The listing builds one solid part. Answer for the finished solid, in the listing's coordinates (mm). Face numbers are marked on the shaded views. A direction names the side the tool comes from. Coordinates: 2 decimals unless noted, no trailing zeros. Order: outer loops, then holes, each group sorted by start corner. A loop starts at its lowest first (then second) coordinate and runs counter-clockwise, first axis right, second up. Notation, with made-up numbers: (-18.75, -26.75) - (36.25, -26.75) arc R22 ccw to (36.25, 10.25) - close; hole circle Ø11 at (14, 81). An arc over 180 degrees is marked (long way). Use one line per item in the form item = value. Start each with the question number.
Item 1: Section A-A, the plane x = 250.5 is taken. Write down the section's boundary in (y, z).
Item 2: Section C-C, the plane x = -10 is taken. Write down the section's boundary in (y, z), and give its area (3 significant figures).
Item 3: Section D-D, the plane z = 117 is taken. Write down the section's boundary in (x, y), and give its area (3 significant figures).
Item 4: A tool of negligible diameter and unlimited length cuts with its end or side. For the marked faces 1 and 2, from which of +Z, -Z, +X, -X, +Y, -Y can it reach the whole face along a straight path? Write none if from no direction.
Item 5: Each of these flat-tipped pins is pushed along its axis until it touches: pin 1 Ø10 at (y, z) = (631.5, 111) entering from -X; pin 2 Ø8 at (x, z) = (366, 13.5) entering from -Y; pin 3 Ø6 at (y, z) = (89.5, 49.5) entering from -X. Where does it stop, or does it pass through?
Item 6: Section B-B, the plane z = 54.5 is taken. Write down the section's boundary in (x, y).
Item 7: The mould has two halves that part along Y. Classify the marked faces 3, 4 and 5: released by +Y, released by -Y, zero draft, split by the parting line, or undercut.
Item 8: Consider line 1 along Y through (x, z) = (99, 37.5); line 2 along X through (y, z) = (195, 49); line 3 along X through (y, z) = (688.5, 42.5). Determine where each line is inside the solid, lowest interval first. Write a range as [from, to].
Autodesk Inventor part; units mm, degrees
ref_plane "YZ Plane" through (0, 0, 0) normal (1, 0, 0) x (0, 1, 0)
ref_plane "XZ Plane" through (0, 0, 0) normal (0, 1, 0) x (-1, 0, 0)
ref_plane "XY Plane" through (0, 0, 0) normal (0, 0, 1) x (1, 0, 0)
sketch "Sketch1" plane through (0, 0, 0) normal (0, 0, 1) x (1, 0, 0)
  line L0 (0, 0) -> (351.6706, 0)
  line L1 (-103.5647, 179.3793) -> (0, 0)
  line L2 (351.6706, 0) -> (455.2353, 179.3793)
  line L3 (455.2353, 179.3793) -> (455.2353, 534.9793)
  line L4 (-103.5647, 534.9793) -> (-103.5647, 179.3793)
  line L5 (0, 714.3586) -> (-103.5647, 534.9793)
  line L6 (356.3091, 714.3586) -> (0, 714.3586)
  line L7 (455.2353, 534.9793) -> (356.3091, 714.3586)
  line L8 (-103.5647, 179.3793) -> (-192.4647, 179.3793) construction
  line L9 (-51.7823, 89.6897) -> (-128.772, 45.2397) construction
  line L10 (-128.772, 45.2397) -> (-51.7823, -88.9)
  line L11 (-51.7823, -88.9) -> (0, -88.9)
  line L12 (178.1545, -88.9) -> (178.1545, 714.3586) construction
  line L13 (178.1545, -88.9) -> (0, -88.9)
  line L14 (-128.772, 45.2397) -> (-192.4647, 156.2119)
  line L15 (-192.4647, 156.2119) -> (-192.4647, 179.3793)
  line L16 (178.1545, 714.3586) -> (178.1545, 803.2586) construction
  line L17 (-51.7823, 624.669) -> (-128.772, 669.119) construction
  line L18 (-192.4647, 179.3793) -> (-192.4647, 558.8)
  line L19 (-192.4647, 558.8) -> (-128.772, 669.119)
  line L20 (178.1545, 803.2586) -> (-51.3264, 803.2586)
  line L21 (-51.3264, 803.2586) -> (-128.772, 669.119)
  line L22 (485.0811, 45.2397) -> (408.0914, -88.9)
  line L23 (178.1545, -88.9) -> (356.3091, -88.9)
  line L24 (485.0811, 45.2397) -> (548.7738, 156.2119)
  line L25 (548.7738, 156.2119) -> (548.7738, 179.3793)
  line L26 (408.0914, 624.669) -> (485.0811, 669.119) construction
  line L27 (548.7738, 179.3793) -> (548.7738, 558.8)
  line L28 (548.7738, 558.8) -> (485.0811, 669.119)
  line L29 (178.1545, 803.2586) -> (407.6355, 803.2586)
  line L30 (407.6355, 803.2586) -> (485.0811, 669.119)
  line L31 (408.0914, -88.9) -> (356.3091, -88.9)
  point P0 (175.8353, 357.1793)
  dimension "d0" = 88.9
  dimension "d1" = 88.9
  dimension "d2" = 88.9
  dimension "d3" = 88.9
  dimension "d4" = 88.9
  dimension "d8" = 88.9
extrude "Extrusion1" add sketch "Sketch1" along normal blind 127
fillet "Fillet1" radius 31.75 24 edges at (63.414, 803.2586, 127) (446.3583, 736.1888, 127) (548.7738, 369.0897, 127) (516.9274, 100.7258, 127) (89.0773, -88.9, 127) (-90.2772, -21.8302, 127) (-192.4647, 167.7956, 127) (-160.6184, 613.9595, 127) (548.7738, 369.0897, 0) (516.9274, 613.9595, 0) (63.414, 803.2586, 0) (-160.6184, 613.9595, 0) (-192.4647, 167.7956, 0) (-90.2772, -21.8302, 0) (-25.8912, -88.9, 0) (446.5863, -21.8302, 0) (548.7738, 156.2119, 63.5) (548.7738, 558.8, 63.5) (407.6355, 803.2586, 63.5) (-51.3264, 803.2586, 63.5) (-192.4647, 558.8, 63.5) (-192.4647, 156.2119, 63.5) (-51.7823, -88.9, 63.5) (408.0914, -88.9, 63.5)
properties part number "Bumpers"
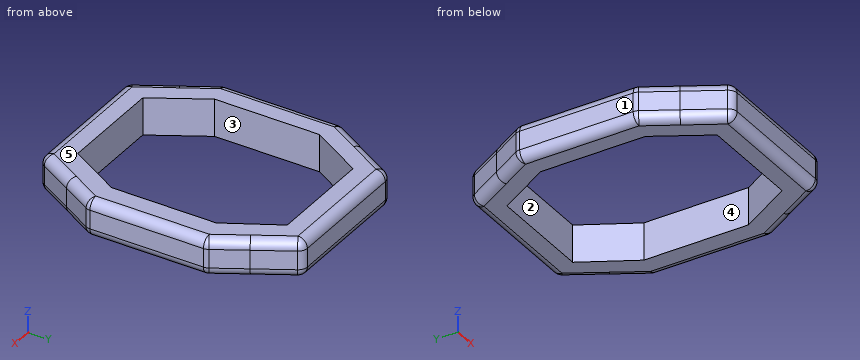
Response:
q1.outline = (-88.9, 31.75) arc R31.75 ccw to (-57.15, 0) - (0, 0) - (0, 127) - (-57.15, 127) arc R31.75 ccw to (-88.9, 95.25) - close; (714.36, 0) - (771.51, 0) arc R31.75 ccw to (803.26, 31.75) - (803.26, 95.25) arc R31.75 ccw to (771.51, 127) - (714.36, 127) - close
q2.outline = (-88.9, 31.75) arc R31.75 ccw to (-57.15, 0) - (17.32, 0) - (17.32, 127) - (-57.15, 127) arc R31.75 ccw to (-88.9, 95.25) - close; (697.04, 0) - (771.51, 0) arc R31.75 ccw to (803.26, 31.75) - (803.26, 95.25) arc R31.75 ccw to (771.51, 127) - (697.04, 127) - close
q2.area = 26,100 mm2
q3.outline = (-183.84, 164.68) arc R23.13 ccw to (-180.78, 153.16) - (-121.3, 49.53) - (-53.46, -68.66) arc R23.13 ccw to (-33.4, -80.28) - (389.71, -80.28) arc R23.13 ccw to (409.77, -68.66) - (477.61, 49.53) - (537.08, 153.16) arc R23.13 ccw to (540.15, 164.68) - (540.15, 550.29) arc R23.13 ccw to (537.06, 561.86) - (477.62, 664.81) - (409.34, 783.07) arc R23.13 ccw to (389.3, 794.64) - (-33, 794.64) arc R23.13 ccw to (-53.03, 783.07) - (-121.31, 664.81) - (-180.75, 561.86) arc R23.13 ccw to (-183.84, 550.29) - close; hole (-103.56, 179.38) - (0, 0) - (351.67, 0) - (455.24, 179.38) - (455.24, 534.98) - (356.31, 714.36) - (0, 714.36) - (-103.56, 534.98) - close
q3.area = 205,000 mm2
q4.face_1 = +Z, -Z, -X, +Y, -Y
q4.face_2 = +Z, -Z
q5.pin_1 = -149.72
q5.pin_2 = -85.52
q5.pin_3 = -155.9
q6.outline = (-192.46, 164.68) arc R31.75 ccw to (-188.25, 148.87) - (-128.77, 45.24) - (-60.93, -72.95) arc R31.75 ccw to (-33.4, -88.9) - (389.71, -88.9) arc R31.75 ccw to (417.24, -72.95) - (485.08, 45.24) - (544.56, 148.87) arc R31.75 ccw to (548.77, 164.68) - (548.77, 550.29) arc R31.75 ccw to (544.52, 566.17) - (485.08, 669.12) - (416.8, 787.38) arc R31.75 ccw to (389.3, 803.26) - (-33, 803.26) arc R31.75 ccw to (-60.49, 787.38) - (-128.77, 669.12) - (-188.21, 566.17) arc R31.75 ccw to (-192.46, 550.29) - close; hole (-103.56, 179.38) - (0, 0) - (351.67, 0) - (455.24, 179.38) - (455.24, 534.98) - (356.31, 714.36) - (0, 714.36) - (-103.56, 534.98) - close
q7.face_3 = undercut
q7.face_4 = undercut
q7.face_5 = zero draft
q8.line_1 = [-88.9, 0], [714.36, 803.26]
q8.line_2 = [-192.46, -103.56], [455.24, 548.77]
q8.line_3 = [-117.58, -14.93], [370.57, 473.89]
